Design review of the part built by this model. Coordinates are the model's own, in mm. Face numbers are marked on the shaded views. A direction names the side the tool comes from. Give positions to 0.01 mm unless a question says otherwise; leave off trailing zeros. Loops run counter-clockwise (first coordinate to the right, second up) from the corner with the lowest first, then second, coordinate; pieces in that order, holes last. Notation, with made-up numbers: (9, 24) -> (47, 24) arc R30 cw to (47, 61) -> close; hole circle Ø11 at (66.25, -34.5). An arc over 180 degrees is marked (long way). Answer in a Markdown table with one row per item. Add a question column.
(1) For pin 1 (6 mm diameter, centred on x = 8, y = -8.5, fed in from +Z); pin 2 (9.5 mm diameter, centred on x = -22, z = -3.5, fed in from -Y); pin 3 (1.5 mm diameter, centred on y = -69.5, z = 0.5, fed in from +X); pin 4 (8 mm diameter, centred on x = -30, y = -92.5, fed in from +Z), all flat-tipped, find the tip position at first contact; note any pin that passes through.
(2) Consider section B-B on x = 8. Count the separate pieces of the cut face and the enclosed holes in it, then the cut area to 3 significant figures.
(3) Consider section A-A on z = -13. Write out the cut boundary in (x, y), then the cut area to 3 significant figures.
(4) Consider section C-C on z = 4. Write out the cut boundary in (x, y), then the cut area to 3 significant figures.
(5) For line 1 (Y direction, x = 8, z = -0.15); line 2 (Z direction, x = 35, y = -61); line 3 (Y direction, x = -19, z = -12), list the stretches that pass through material, from the lowest coordinate up.
(6) For the marked faces 1, 2 and 3, list the 3-axis set-ups (+Z, -Z, +X, -X, +Y, -Y) from which the entire face can be reached by the end or side of a thin tool; tool diameter is ignored.
from build123d import *

# Parameters (mm, degrees)
CROQUIS1_W              = 100
CROQUIS1_H              = 31
SALIENTE_EXTRUIR1_DEPTH = 2.5
CROQUIS2_W              = 92
CROQUIS2_H              = 15
SALIENTE_EXTRUIR2_DEPTH = 3
REDONDEO1_R             = 5
SALIENTE_EXTRUIR3_DEPTH = 2.5
CROQUIS4_R              = 2.25
CORTAR_EXTRUIR1_DEPTH   = 5
CROQUIS5_W              = 11
CROQUIS5_H              = 2.5
CORTAR_EXTRUIR2_DEPTH   = 32


with BuildPart() as part:
    # Croquis1 → Saliente-Extruir1 (new body)
    with BuildSketch(Plane(origin=(0, 0, 0), x_dir=(1, 0, 0), z_dir=(0, 1, 0))):
        Rectangle(CROQUIS1_W, CROQUIS1_H)
    extrude(amount=SALIENTE_EXTRUIR1_DEPTH)

    # Croquis2 → Saliente-Extruir2 (add)
    with BuildSketch(Plane.XZ):
        with Locations((4, 0)):
            Rectangle(CROQUIS2_W, CROQUIS2_H)
    extrude(amount=SALIENTE_EXTRUIR2_DEPTH)

    # Redondeo1
    redondeo1_edges = [part.edges().sort_by_distance(p)[0] for p in [
        (50, -1.5, -7.5),
        (50, -1.5, 7.5),
        (-42, -1.5, 7.5),
        (-42, -1.5, -7.5),
        (50, 1.25, 15.5),
        (-50, 1.25, 15.5),
        (-50, 1.25, -15.5),
        (50, 1.25, -15.5),
    ]]
    fillet(redondeo1_edges, radius=REDONDEO1_R)

    # Croquis3 → Saliente-Extruir3 (add, symmetric)
    with BuildSketch(Plane.XY):
        with BuildLine():
            Line((50.268673777, -3), (-42, -3))
            add(Edge.make_bspline(
                [(-42, -3), (-40.908513064, -23.29428707), (-48.776278563, -61.439241492), (-15.011612903, -108.496757753), (26.091280983, -116.271998862), (53.921744721, -120.172870924), (68.330972256, -122.076661229), (72.745319056, -119.457978538)],
                knots=[0, 0, 0, 0, 0.313172426, 0.560686791, 0.787562365, 0.924725026, 1, 1, 1, 1], degree=3))
            add(Edge.make_bspline(
                [(72.745319056, -119.457978538), (73.5272978, -115.295050348), (67.866383472, -111.564174063), (40.837413629, -79.656102563), (38.369873508, -37.789508287), (50.268673777, -3)],
                knots=[0, 0, 0, 0, 0.326988998, 0.554852248, 1, 1, 1, 1], degree=3))
        make_face()
    extrude(amount=SALIENTE_EXTRUIR3_DEPTH, both=True)

    # Croquis4 → Cortar-Extruir1 (cut)
    with BuildSketch(Plane.XY.offset(2.5)):
        with Locations((8, -8.5)):
            Circle(CROQUIS4_R)
        with Locations((8, -98.5)):
            Circle(CROQUIS4_R)
    extrude(amount=-CORTAR_EXTRUIR1_DEPTH, mode=Mode.SUBTRACT)

    # Croquis5 → Cortar-Extruir2 (cut, through all)
    with BuildSketch(Plane.XY.offset(15.5)):
        with Locations((-4.5, 1.25)):
            Rectangle(CROQUIS5_W, CROQUIS5_H)
    extrude(amount=-CORTAR_EXTRUIR2_DEPTH, mode=Mode.SUBTRACT)


solid = part.part
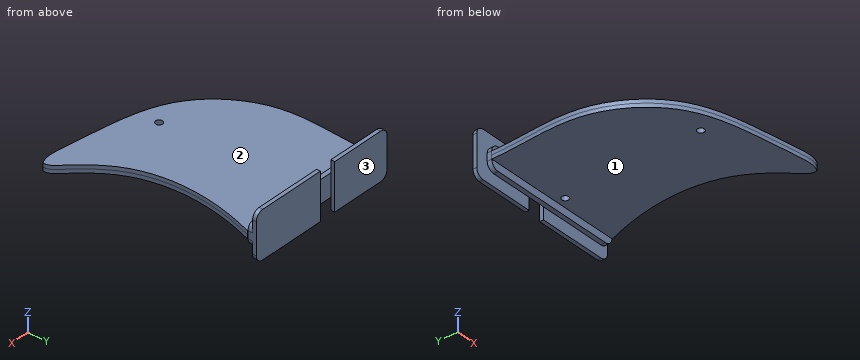
Values follow:
| question | item | result |
|---|---|---|
| 1 | pin 1 | z = 2.5 |
| 1 | pin 2 | y = -99.01 |
| 1 | pin 3 | x = 43.89 |
| 1 | pin 4 | through |
| 2 | separate pieces | 3 |
| 2 | enclosed holes | 0 |
| 2 | area | 622 mm2 |
| 3 | outline | (-49.33, 0) -> (-10, 0) -> (-10, 2.5) -> (-49.33, 2.5) -> close; (1, 0) -> (49.33, 0) -> (49.33, 2.5) -> (1, 2.5) -> close |
| 3 | area | 219 mm2 |
| 4 | outline | (-50, 0) -> (-41.77, 0) -> (-41.77, -3) -> (49.77, -3) -> (49.77, 0) -> (50, 0) -> (50, 2.5) -> (1, 2.5) -> (1, 0) -> (-10, 0) -> (-10, 2.5) -> (-50, 2.5) -> close |
| 4 | area | 497 mm2 |
| 5 | line 1 | -111.95 to -100.75, -96.25 to -10.75, -6.25 to 2.5 |
| 5 | line 2 | -2.5 to 2.5 |
| 5 | line 3 | 0 to 2.5 |
| 6 | face 1 | -Z, +X, -X, -Y |
| 6 | face 2 | +Z, +X, -X, -Y |
| 6 | face 3 | +Z, -Z, +X, -X, +Y |
